Part model, mm, in its own coordinate system. Give positions to 0.01 mm unless a question says otherwise; leave off trailing zeros. Order: outer loops, then holes, each group sorted by start corner. A loop starts at its lowest first (then second) coordinate and runs counter-clockwise, first axis right, second up. Notation, with made-up numbers: (27, 24.5) -> (81, 24.5) arc R12 ccw to (81, 30.5) -> close; hole circle Ø10 at (44, 20). An arc over 180 degrees is marked (long way). Write item = value, one per line. Start each with the question number.
(1) Probe line 1 along X through (y, z) = (2.75, 0.3); line 2 along Y through (x, z) = (36.5, 2.25); line 3 along Y through (x, z) = (11, -1.65). List the from-to ranges inside material, lowest first. Write a range as from..to.
(2) Flat gauge pin, fed straight in: pin 1 (1 mm diameter, centred on x = 34, z = -0.5, fed in from -Y). Where does the tip first touch, or does it go through?
(3) Saw through at B-B, the plane x = -4.5. List the corners of the cut face in (y, z).
(4) Saw through at A-A, the plane y = 2. List the corners of the cut face in (x, z), then the cut area to 4 significant figures.
from build123d import *

# Parameters (mm, degrees)
SKETCH1_W                       = 86
SKETCH1_H                       = 5
BOSS_EXTRUDE1_DEPTH             = 6.2
SKETCH2_W                       = 7.35
SKETCH2_H                       = 4.7
CUT_EXTRUDE1_DEPTH              = 10
SKETCH3_R                       = 0.5
FIRST_HOLD_DOWN_CYLINDERS_DEPTH = 1
LPATTERN1_COUNT                 = 5
LPATTERN1_PITCH                 = 9
LPATTERN1_COL_COUNT             = 4
LPATTERN1_COL_PITCH             = 9
FIRST_RIDGE_DEPTH               = 7.35
RACK_LEFT_PATTERN_COUNT         = 4
RACK_LEFT_PATTERN_PITCH         = 0.66294
RACK_LEFT_PATTERN_COL_COUNT     = 4
RACK_LEFT_PATTERN_COL_PITCH     = 0.66
MIRROR2_COPY_1_DEPTH            = 7.35
MIRROR2_COPY_2_DEPTH            = 7.35
MIRROR2_COPY_3_DEPTH            = 7.35
MIRROR2_COPY_4_DEPTH            = 7.35
MIRROR2_COPY_5_DEPTH            = 7.35
MIRROR2_COPY_6_DEPTH            = 7.35


with BuildPart() as part:
    # Sketch1 → Boss-Extrude1 (new body)
    with BuildSketch(Plane(origin=(0, 0, 0), x_dir=(1, 0, 0), z_dir=(0, 1, 0))):
        Rectangle(SKETCH1_W, SKETCH1_H)
    extrude(amount=BOSS_EXTRUDE1_DEPTH)

    # Sketch2 → Cut-Extrude1 (cut)
    with BuildSketch(Plane.XY.offset(2.5)):
        with Locations((39.325, 2.35)):
            Rectangle(SKETCH2_W, SKETCH2_H)
    cut_extrude1 = extrude(amount=-CUT_EXTRUDE1_DEPTH, mode=Mode.SUBTRACT)

    # Mirror1: Cut-Extrude1 across plane
    add(cut_extrude1.mirror(Plane(origin=(0, 0, 0), x_dir=(0, 0, 1), z_dir=(1, 0, 0))), mode=Mode.SUBTRACT)

    # Sketch3 → First hold-down cylinders (add)
    with BuildSketch(Plane.XZ):
        with Locations(Location((-3, 0, 0), (0, 0, 90))):
            Circle(SKETCH3_R)
        with Locations(Location((-6, 0, 0), (0, 0, 90))):
            Circle(SKETCH3_R)
    first_hold_down_cylinders = extrude(amount=FIRST_HOLD_DOWN_CYLINDERS_DEPTH)

    # LPattern1: First hold-down cylinders ×5
    with Locations(*[(i * LPATTERN1_PITCH, 0, 0) for i in range(1, LPATTERN1_COUNT)]):
        add(first_hold_down_cylinders)

    # LPattern1 col: First hold-down cylinders ×4
    with Locations(*[(-i * LPATTERN1_COL_PITCH, 0, 0) for i in range(1, LPATTERN1_COL_COUNT)]):
        add(first_hold_down_cylinders)

    # Sketch4 → First Ridge (add)
    with BuildSketch(Plane(origin=(43, 0, 0), x_dir=(0, 0, -1), z_dir=(1, 0, 0))):
        Polygon((0.220588094, 4.7), (-0.220588094, 4.7), (-0.075, 4.3), (0.075, 4.3), align=None)
    first_ridge = extrude(amount=-FIRST_RIDGE_DEPTH)

    # Rack Left Pattern: First Ridge ×4
    with Locations(*[(0, 0, i * RACK_LEFT_PATTERN_PITCH) for i in range(1, RACK_LEFT_PATTERN_COUNT)]):
        add(first_ridge)

    # Rack Left Pattern col: First Ridge ×4
    with Locations(*[(0, 0, -i * RACK_LEFT_PATTERN_COL_PITCH) for i in range(1, RACK_LEFT_PATTERN_COL_COUNT)]):
        add(first_ridge)

    # Mirror2: First Ridge across plane
    add(first_ridge.mirror(Plane(origin=(0, 0, 0), x_dir=(0, 0, 1), z_dir=(1, 0, 0))))

    # Mirror2 copy 1 sketch → Mirror2 copy 1 (add)
    with BuildSketch(Plane(origin=(-43, 0, 0.66294), x_dir=(0, 0, -1), z_dir=(-1, 0, 0))):
        Polygon((0.220588094, -4.7), (-0.220588094, -4.7), (-0.075, -4.3), (0.075, -4.3), align=None)
    extrude(amount=-MIRROR2_COPY_1_DEPTH)

    # Mirror2 copy 2 sketch → Mirror2 copy 2 (add)
    with BuildSketch(Plane(origin=(-43, 0, 1.32588), x_dir=(0, 0, -1), z_dir=(-1, 0, 0))):
        Polygon((0.220588094, -4.7), (-0.220588094, -4.7), (-0.075, -4.3), (0.075, -4.3), align=None)
    extrude(amount=-MIRROR2_COPY_2_DEPTH)

    # Mirror2 copy 3 sketch → Mirror2 copy 3 (add)
    with BuildSketch(Plane(origin=(-43, 0, 1.98882), x_dir=(0, 0, -1), z_dir=(-1, 0, 0))):
        Polygon((0.220588094, -4.7), (-0.220588094, -4.7), (-0.075, -4.3), (0.075, -4.3), align=None)
    extrude(amount=-MIRROR2_COPY_3_DEPTH)

    # Mirror2 copy 4 sketch → Mirror2 copy 4 (add)
    with BuildSketch(Plane(origin=(-43, 0, -0.66), x_dir=(0, 0, -1), z_dir=(-1, 0, 0))):
        Polygon((0.220588094, -4.7), (-0.220588094, -4.7), (-0.075, -4.3), (0.075, -4.3), align=None)
    extrude(amount=-MIRROR2_COPY_4_DEPTH)

    # Mirror2 copy 5 sketch → Mirror2 copy 5 (add)
    with BuildSketch(Plane(origin=(-43, 0, -1.32), x_dir=(0, 0, -1), z_dir=(-1, 0, 0))):
        Polygon((0.220588094, -4.7), (-0.220588094, -4.7), (-0.075, -4.3), (0.075, -4.3), align=None)
    extrude(amount=-MIRROR2_COPY_5_DEPTH)

    # Mirror2 copy 6 sketch → Mirror2 copy 6 (add)
    with BuildSketch(Plane(origin=(-43, 0, -1.98), x_dir=(0, 0, -1), z_dir=(-1, 0, 0))):
        Polygon((0.220588094, -4.7), (-0.220588094, -4.7), (-0.075, -4.3), (0.075, -4.3), align=None)
    extrude(amount=-MIRROR2_COPY_6_DEPTH)


solid = part.part
Results list:
q1.line_1 = -35.65..35.65
q1.line_2 = 4.7..6.2
q1.line_3 = 0..6.2
q2.pin_1 = 0
q3.outline = (0, -2.5) -> (6.2, -2.5) -> (6.2, 2.5) -> (0, 2.5) -> close
q4.outline = (-35.65, -2.5) -> (35.65, -2.5) -> (35.65, 2.5) -> (-35.65, 2.5) -> close
q4.area = 356.5 mm^2
